Geometry check sheet. Reference: the model listing, model coordinates, mm. Face numbers are marked on the shaded views. A direction names the side the tool comes from. Coordinates: 2 decimals unless noted, no trailing zeros. Order: outer loops, then holes, each group sorted by start corner. A loop starts at its lowest first (then second) coordinate and runs counter-clockwise, first axis right, second up. Notation, with made-up numbers: (63, 32.5) - (96, 32.5) arc R23 ccw to (96, 49.5) - close; hole circle Ø6 at (14, -14.5). An arc over 180 degrees is marked (long way). One line per item, written item: value. Start each with the question number.
Autodesk Inventor part; units mm, degrees
ref_plane "Work Plane1" through (0, 2, 0) normal (0, 1, 0) x (-1, 0, 0)
ref_plane "YZ Plane" through (0, 0, 0) normal (1, 0, 0) x (0, 1, 0)
ref_plane "XY Plane" through (0, 0, 0) normal (0, 0, 1) x (1, 0, 0)
sketch "Sketch1" plane through (0, 0, 0) normal (0, 0, 1) x (1, 0, 0)
  line L0 (5, 0) -> (6.45, 0)
  line L1 (0, 13) -> (0, 11.4819)
  line L2 (6, 1) -> (6.45, 1)
  line L3 (6, 1.8) -> (6.45, 1.8)
  line L4 (6, 1.8) -> (6, 1)
  line L5 (6.45, 0) -> (6.45, 1)
  line L6 (6, 7) -> (6.45, 7)
  line L7 (6, 7.8) -> (6.45, 7.8)
  line L8 (6, 7.8) -> (6, 7)
  line L9 (6.45, 1.8) -> (6.45, 7)
  line L10 (6, 9) -> (6.45, 9)
  line L11 (6, 9.8) -> (6.45, 9.8)
  line L12 (6, 9.8) -> (6, 9)
  line L13 (6.45, 7.8) -> (6.45, 9)
  line L14 (6.45, 9.8) -> (6.45, 11)
  line L15 (0, 13) -> (6.45, 11)
  line L16 (5, 9.9315) -> (5, 0)
  line L17 (0, 11.4819) -> (5, 9.9315)
  point P0 (0, 0)
revolve "Revolution1" add sketch "Sketch1" angle 360 about axis through (0, 13, 0) along (0, -1, 0)
ref_plane "Work Plane1" through (0, 2, 0) normal (0, 1, 0) x (-1, 0, 0)
sketch "Sketch2" plane through (0, 2, 0) normal (0, 1, 0) x (-1, 0, 0)
  line L0 (-3, 2.5) -> (-3, -2.5)
  line L1 (3, 2.5) -> (3, -2.5)
  line L2 (4.3301, 2.5) -> (3, 2.5)
  line L3 (-3, 2.5) -> (-4.3301, 2.5)
  line L4 (4.3301, -2.5) -> (3, -2.5)
  line L5 (-3, -2.5) -> (-4.3301, -2.5)
  arc A0 (-4.3301, 2.5) -> (-4.3301, -2.5) centre (0, 0) ccw
  arc A1 (4.3301, -2.5) -> (4.3301, 2.5) centre (0, 0) ccw
extrude "Extrusion1" add sketch "Sketch2" along normal blind 9
fillet "Fillet1" radius 2.5 4 edges at (-3.6651, 2, 2.5) (-3.6651, 2, -2.5) (3.6651, 2, 2.5) (3.6651, 2, -2.5)
sketch "Sketch3" plane through (0, 0, 0) normal (1, 0, 0) x (0, 1, 0)
  circle A0 centre (5, 0) radius 1.5
extrude "Extrusion2" cut sketch "Sketch3" along normal mid plane 20
properties part number "piston"
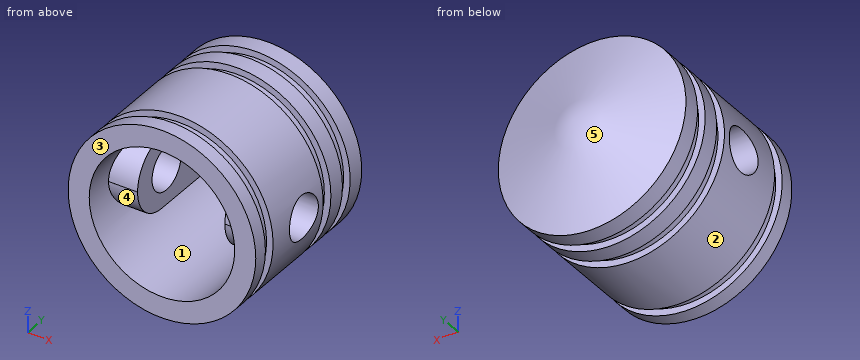
Q1. Set-up check for the marked faces 4 and 5: record each of +Z, -Z, +X, -X, +Y, -Y from which the full face is reachable in a straight line by a thin tool's end or side.
Q2. Cross-section at A-A, the plane y = 2.5. Enter the section's corners in (x, z), and give its area (3 significant figures).
Q3. Material ranges on probe 1 along Z at (x, y) = (-3.75, 6.75); probe 2 along Z at (x, y) = (-2.25, 8); probe 3 along Z at (x, y) = (-1.75, 3.5), recorded low to high.
Q4. Cross-section at C-C, the plane z = -1. Count the separate pieces of the cut face and the enclosed holes in it, and give its area (3 significant figures).
Q5. Release check for a two-part mould opening along Z. For the marked faces 1, 2 and 3 record: released by +Z, released by -Z, zero draft, split by the parting line, or undercut.
Q6. Cross-section at B-B, the plane y = 5. Enter the section's corners in (x, z), and give its area (3 significant figures).
Q7. Cross-section at D-D, the plane y = 12. Enter the section's corners in (x, z) (3 decimals).
Q8. Gauge pin test, flat ends, axial feed: P1, Ø4, axis at x = -1.5, z = -1.5, coming from the -Y side; P2, Ø1.1, axis at x = -4, y = 7, coming from the +Z side; P3, Ø1.1, axis at x = -3.5, y = 6, coming from the -Z side. Record the tip position at first contact, or that the pin passes through.
Check result:
1. face 4: -Y
1. face 5: +Y
2. outline: circle Ø12.9 at (0, 0); hole (-4.77, -1.5) arc R5 ccw to (4.77, -1.5) - (3, -1.5) - (3, 1.5) - (4.77, 1.5) arc R5 ccw to (-4.77, 1.5) - (-3, 1.5) - (-3, -1.5) - close
2. area: 63.7 mm2
3. probe 1: z = -5.25 to -3.31, -2.5 to 2.5, 3.31 to 5.25
3. probe 2: z = -6.04 to -4.47, 4.47 to 6.04
3. probe 3: z = -6.21 to -4.68, 4.68 to 6.21
4. separate pieces: 3
4. enclosed holes: 0
4. area: 61.1 mm2
5. face 1: undercut
5. face 2: split by the parting line
5. face 3: zero draft
6. outline: (-6.27, -1.5) arc R6.45 ccw to (6.27, -1.5) - (3, -1.5) - (3, -2.5) - (4.33, -2.5) arc R5 cw to (-4.33, -2.5) - (-3, -2.5) - (-3, -1.5) - close; (-6.27, 1.5) - (-3, 1.5) - (-3, 2.5) - (-4.33, 2.5) arc R5 cw to (4.33, 2.5) - (3, 2.5) - (3, 1.5) - (6.27, 1.5) arc R6.45 ccw to start
6. area: 49.6 mm2
7. outline: circle Ø6.45 at (0, 0)
8. P1: stops at y = 2.01
8. P2: stops at z = 5.45
8. P3: stops at z = -5.74
